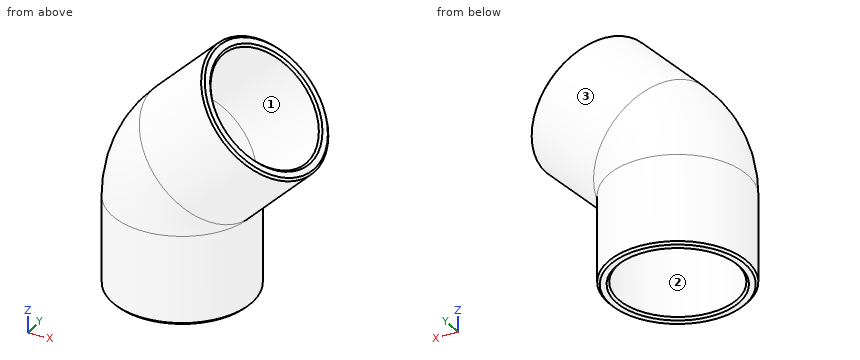
```python
from build123d import *

# Parameters (mm, degrees)
F2_R     = 24.765
F2_R_2   = 21.082
F4_SIZE  = 0.7874
F5_SCALE = 1.45


with BuildPart() as f3:
    # F3: sweep along a path in F0
    with BuildLine(Plane.XZ) as f3_path:
        Line((0, -42.0079988722), (0, -10.3106039946))
        ThreePointArc((0, -10.3106039946), (1.8947906767, -0.7848479962), (7.2906980027, 7.2906980027))
        Line((7.2906980027, 7.2906980027), (29.7041408666, 29.7041408666))
    # F2 (on plane+point) → F3 (sweep)
    with BuildSketch(Plane.XY.offset(-42.0079988722)):
        Circle(F2_R)
        Circle(F2_R_2, mode=Mode.SUBTRACT)
    sweep(path=f3_path.line)

    # F4
    f4_edges = [f3.edges().sort_by_distance(p)[0] for p in [
        (12.192641, 0, 47.21564),
        (14.796916, 0, 44.611366),
        (-21.082, 0, -42.007999),
        (-24.765, 0, -42.007999),
    ]]
    chamfer(f4_edges, length=F4_SIZE)


with BuildPart() as f3_1:
    # F5: moved
    add(f3.part.scale(F5_SCALE))


solid = f3_1.part
```
Design review of the part built by this model. Coordinates are the model's own, in mm. Face numbers are marked on the shaded views. Coordinates: 2 decimals unless noted, no trailing zeros. Loops run counter-clockwise (first coordinate to the right, second up) from the corner with the lowest first, then second, coordinate; pieces in that order, holes last.
Q1. We need section B-B on z = -47.5. State the section outline as (x, y) points, and give its area (3 significant figures).
Reported:
outline: circle Ø71.82 at (0, 0); hole circle Ø61.14 at (0, 0)
area: 1,120 mm2
Q2. For pin 1 (12 mm diameter, centred on x = 19, y = 2.5, fed in from -Z); pin 2 (8 mm diameter, centred on x = 43, z = 25.5, fed in from -Y); pin 3 (3 mm diameter, centred on x = 6.5, y = -4.5, fed in from -Z), all flat-tipped, find the tip position at first contact; note any pin that passes through.
Reported:
pin 1: stops at z = 56.03
pin 2: stops at y = -34.92
pin 3: stops at z = 47.72
Q3. We need section A-A on y = 0. State the section outline as (x, z) points, and give its area (3 significant figures).
Reported:
outline: (-35.91, -59.77) - (-34.77, -60.91) - (-31.71, -60.91) - (-30.57, -59.77) - (-30.57, -14.95) arc R66.66 cw to (-11.04, 32.19) - (20.65, 63.88) - (20.65, 65.49) - (18.49, 67.66) - (16.87, 67.66) - (-14.82, 35.96) arc R72 ccw to (-35.91, -14.95) - close; (30.57, -59.77) - (31.71, -60.91) - (34.77, -60.91) - (35.91, -59.77) - (35.91, -14.95) arc R0.18 cw to (35.96, -14.82) - (67.66, 16.87) - (67.66, 18.49) - (65.49, 20.65) - (63.88, 20.65) - (32.19, -11.04) arc R5.52 ccw to (30.57, -14.95) - close
area: 1,280 mm2
Q4. The part is to be moulded in two halves that separate along Y. For the marked faces 1, 2 and 3, say which applies: +Y half, -Y half, draft (parallel to the pull), parting line (faces both ways), or undercut.
Reported:
face 1: undercut
face 2: undercut
face 3: parting line
Q5. To check wall thickness, follow line 1 (Y direction, x = 0, z = -40); line 2 (Y direction, x = 29, z = 27); line 3 (Z direction, x = 26, y = 26). State the ranges of each line that lie inside material, in increasing order.
Reported:
line 1: y = -35.91 to -30.57, 30.57 to 35.91
line 2: y = -35.88 to -30.54, 30.54 to 35.88
line 3: z = -9.81 to 3.26, 48.74 to 59.54
